```python
from build123d import *

# Parameters (mm, degrees)
BOSS_EXTRUDE1_DEPTH = 21
SKETCH2_R           = 71
SKETCH2_R_2         = 41.5
BOSS_EXTRUDE2_DEPTH = 2
SKETCH3_W           = 50
SKETCH3_H           = 20
BOSS_EXTRUDE3_DEPTH = 15
SKETCH8_R           = 1.6
BOSS_EXTRUDE5_DEPTH = 5
FILLET2_R           = 15
SKETCH11_W          = 43.237900078
SKETCH11_H          = 3
CUT_EXTRUDE7_DEPTH  = 20
SKETCH12_R          = 1.7
CUT_EXTRUDE8_DEPTH  = 10


with BuildPart() as part:
    # Sketch1 → Boss-Extrude1 (new body)
    with BuildSketch(Plane.XY):
        with BuildLine():
            Line((71, 0), (70, 0))
            ThreePointArc((70, 0), (0, -70), (-70, 0))
            Line((-70, 0), (-71, 0))
            ThreePointArc((-71, 0), (0, -71), (71, 0))
        make_face()
    extrude(amount=BOSS_EXTRUDE1_DEPTH)

    # Sketch2 → Boss-Extrude2 (add)
    with BuildSketch(Plane.XY.offset(21)):
        Circle(SKETCH2_R)
        Circle(SKETCH2_R_2, mode=Mode.SUBTRACT)
    extrude(amount=BOSS_EXTRUDE2_DEPTH)

    # Sketch3 → Boss-Extrude3 (add)
    with BuildSketch(Plane(origin=(0, 0, 0), x_dir=(-1, 0, 0), z_dir=(0, 0, -1))):
        with BuildLine():
            Line((-25, -66.452990903), (-25, -71))
            Line((-25, -71), (0, -71))
            ThreePointArc((0, -71), (-12.705070757, -69.853999006), (-25, -66.452990903))
        make_face()
        with BuildLine():
            ThreePointArc((25, -66.452990903), (12.705070757, -69.853999006), (0, -71))
            Line((0, -71), (25, -71))
            Line((25, -71), (25, -66.452990903))
        make_face()
        with Locations((0, -81)):
            Rectangle(SKETCH3_W, SKETCH3_H)
    extrude(amount=-BOSS_EXTRUDE3_DEPTH)

    # Sketch8 → Boss-Extrude5 (add)
    # profile 1 of 2: a face of its own
    with BuildSketch(Plane(origin=(0, 0, 0), x_dir=(-1, 0, 0), z_dir=(0, 0, -1))):
        with BuildLine():
            ThreePointArc((-70.654086931, -7), (-70.913469003, -3.504270818), (-71, 0))
            Line((-71, 0), (-78, 0))
            Line((-78, 0), (-78, -7))
            Line((-78, -7), (-70.654086931, -7))
        make_face()
        with Locations((-74.5, -3.5)):
            Circle(SKETCH8_R, mode=Mode.SUBTRACT)
    # profile 2 of 2: a face of its own
    with BuildSketch(Plane(origin=(0, 0, 0), x_dir=(-1, 0, 0), z_dir=(0, 0, -1))):
        with BuildLine():
            Line((78, 0), (71, 0))
            ThreePointArc((71, 0), (70.913469003, -3.504270818), (70.654086931, -7))
            Line((70.654086931, -7), (78, -7))
            Line((78, -7), (78, 0))
        make_face()
        with Locations(Location((74.5, -3.5, 0), (0, 0, 180))):
            Circle(SKETCH8_R, mode=Mode.SUBTRACT)
    extrude(amount=-BOSS_EXTRUDE5_DEPTH)

    # Fillet2
    fillet2_edges = [part.edges().sort_by_distance(p)[0] for p in [
        (-25, -78.726495452, 15),
        (25, -78.726495452, 15),
    ]]
    fillet(fillet2_edges, radius=FILLET2_R - 0.0001)  # a hair under: the kernel refuses the full size

    # Sketch11 → Cut-Extrude7 (cut)
    with BuildSketch(Plane.XZ.offset(91)):
        with Locations((0, 1.5)):
            Rectangle(SKETCH11_W, SKETCH11_H)
        with BuildLine():
            Line((-21.618950039, 3), (21.618950039, 3))
            ThreePointArc((21.618950039, 3), (17.348469228, 9.486832981), (10, 12))
            Line((10, 12), (-10, 12))
            ThreePointArc((-10, 12), (-17.348469228, 9.486832981), (-21.618950039, 3))
        make_face()
    extrude(amount=-CUT_EXTRUDE7_DEPTH, mode=Mode.SUBTRACT)

    # Sketch12 → Cut-Extrude8 (cut)
    with BuildSketch(Plane.XY.offset(23)):
        with Locations((0, 60)):
            Circle(SKETCH12_R)
    extrude(amount=-CUT_EXTRUDE8_DEPTH, mode=Mode.SUBTRACT)


solid = part.part
```
The listing builds one solid part. Answer for the finished solid, in the listing's coordinates (mm). A direction names the side the tool comes from. Coordinates: 2 decimals unless noted, no trailing zeros. Loops run counter-clockwise (first coordinate to the right, second up) from the corner with the lowest first, then second, coordinate; pieces in that order, holes last. Notation, with made-up numbers: (79, -39) - (100, -39) arc R14 cw to (100, -30) - close; hole circle Ø2 at (61, -35). An arc over 180 degrees is marked (long way). Use a Markdown table: item, result. Add a question column.
1) The part is cut by section D-D, the plane y = 37. Give the vertices of the cut face in (x, z), and give its area (3 significant figures).
2) The mould has two halves that part along X. Classify faces 1 (the flat face through (73, 0, 4)), 2 (the cylindrical face through (-0.221, 61.686, 22.014)), 3 (the cylindrical face through (20.49, -78.9, 10.72)), 4 (the cylindrical face through (-17.261, -81.14, 9.554)): released by +X, released by -X, zero draft, split by the parting line, or undercut.
3) The part is cut by section A-A, the plane y = -38. Give the vertices of the cut face in (x, z) (3 decimals), and give its area (3 significant figures).
4) The part is cut by section B-B, the plane z = 8. Give the vertices of the cut face in (x, y).
5) The part is cut by section C-C, the plane x = 54.5. Give the vertices of the cut face in (y, z), and give its area (3 significant figures).
6) Find the intervals of material crossed by line 1 (Y direction, x = 0, z = 21.75); line 2 (Y direction, x = -74.5, z = 1.3); line 3 (Z direction, x = 67, y = -3.5), in increasing order.
7) For faces 5 (the cylindrical face through (17.436, -81.14, 9.419)), 6 (the flat face through (-74, -7, 2)), 7 (the flat face through (74, -7, 2)), 8 (the flat face through (31, -30, 21)), determine the directions among +Z, -Z, +X, -X, +Y, -Y from which every point of the face is accessible in a straight line to the end or side of a thin tool.
8) Given pin 1 (8 mm diameter, centred on x = 59, z = 10, fed in from -Y); pin 2 (13 mm diameter, centred on x = 6, z = 4.5, fed in from -Y); pin 3 (1.9 mm diameter, centred on x = 74.5, y = -3.5, fed in from +Z); pin 4 (2.5 mm diameter, centred on y = -82, z = 1, fed in from +X), each flat-ended and moving along its own axis, determine where each tip first touches the part or whether it passes through.
Here are the results:
| question | item | result |
|---|---|---|
| 1 | outline | (-60.6, 21) - (-18.79, 21) - (-18.79, 23) - (-60.6, 23) - close; (18.79, 21) - (60.6, 21) - (60.6, 23) - (18.79, 23) - close |
| 1 | area | 167 mm^2 |
| 2 | face 1 | zero draft |
| 2 | face 2 | undercut |
| 2 | face 3 | released by +X |
| 2 | face 4 | undercut |
| 3 | outline | (-59.975, 0) - (-58.788, 0) - (-58.788, 21) - (-16.681, 21) - (-16.681, 23) - (-59.975, 23) - close; (16.681, 21) - (58.788, 21) - (58.788, 0) - (59.975, 0) - (59.975, 23) - (16.681, 23) - close |
| 3 | area | 223 mm^2 |
| 4 | outline | (-71, 0) arc R71 ccw to (-22.69, -67.28) - (-22.69, -91) - (-18.94, -91) - (-18.94, -71) - (18.94, -71) - (18.94, -91) - (22.69, -91) - (22.69, -67.28) arc R71 ccw to (71, 0) - (70, 0) arc R70 cw to (-70, 0) - close |
| 5 | outline | (-45.51, 0) - (-43.93, 0) - (-43.93, 21) - (45.51, 21) - (45.51, 23) - (-45.51, 23) - close |
| 5 | area | 215 mm^2 |
| 6 | line 1 | y = -71 to -41.5, 41.5 to 58.3, 61.7 to 71 |
| 6 | line 2 | y = -7 to -5.1, -1.9 to 0 |
| 6 | line 3 | z = 21 to 23 |
| 7 | face 5 | -Z, -Y |
| 7 | face 6 | +Z, -Z, -X, -Y |
| 7 | face 7 | +Z, -Z, +X, -Y |
| 7 | face 8 | -Z, +Y |
| 8 | pin 1 | stops at y = -44.9 |
| 8 | pin 2 | stops at y = -71 |
| 8 | pin 3 | passes through |
| 8 | pin 4 | stops at x = 25 |
